CAD build for the part. Positions are in the model's coordinates, mm. Round coordinates to 2 decimals unless told otherwise and drop trailing zeros. Write each loop counter-clockwise with the first axis right and the second up, starting at its lowest first coordinate (ties: lowest second). Pieces come first, ordered by that corner, then holes. Notation, with made-up numbers: (41.5, 81) -> (67.5, 81) arc R14 cw to (67.5, 93) -> close; hole circle Ø8 at (-25, 60). An arc over 180 degrees is marked (long way). Put each result on its own line as item: value. Start each with the question number.
1. Flat gauge pins, fed straight in: P1, Ø8, axis at x = -3039.73, z = -145.15, coming from the +Y side; P2, Ø11.5, axis at x = -2919.73, z = -145.15, coming from the -Y side. Where does each tip first touch, or does it go through?
2. Drill centre lines: line 1 (X direction, y = 17.5, z = -35.5); line 2 (X direction, y = 20, z = -137); line 3 (Z direction, x = -3767.5, y = 2). Where is each one in solid material? Low to high. Write a range as from..to.
3. Saw through at A-A on z = -96. List the corners of the cut face in (x, y).
4. Saw through at B-B on x = -3637. List the corners of the cut face in (y, z).
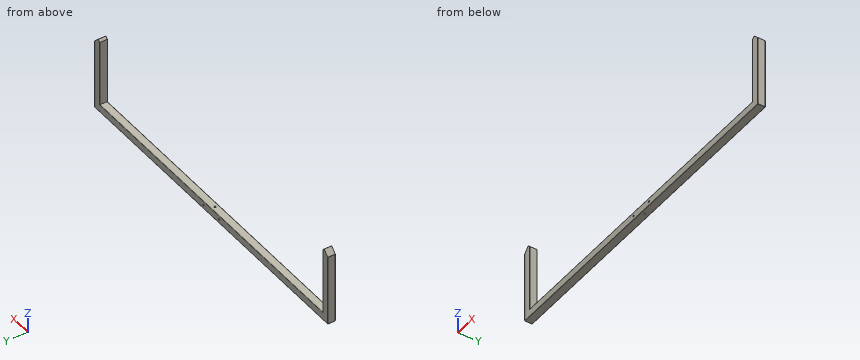
Autodesk Inventor part; units mm, degrees
ref_plane "YZ Plane" through (0, 0, 0) normal (1, 0, 0) x (0, 1, 0)
ref_plane "XZ Plane" through (0, 0, 0) normal (0, 1, 0) x (-1, 0, 0)
ref_plane "XY Plane" through (0, 0, 0) normal (0, 0, 1) x (1, 0, 0)
sketch "Sketch1" plane through (0, 0, 0) normal (0, 1, 0) x (-1, 0, 0)
  line L0 (3880.5632, 208.6837) -> (3853.3913, 235.9005)
  arc A0 (3880.5632, 208.6837) -> (3881.9735, 208.0967) centre (3881.9785, 210.0967) ccw
  line L1 (2078.8655, 206.2751) -> (2106.1695, 233.5659)
  arc A1 (2077.4795, 205.6899) -> (2078.8655, 206.2751) centre (2077.4516, 207.6897) ccw
  arc A2 (3883.0351, 262.7329) -> (3883.0378, 262.7357) centre (2978.5428, 1160.9837) ccw
  arc A3 (3881.9735, 261.6652) -> (3881.9774, 261.6692) centre (2978.5428, 1160.9837) ccw
  line L2 (2979.7274, -125.1538) -> (3881.9735, -125.1538)
  line L3 (3879.7274, -165.1538) -> (2079.7274, -165.1538)
  line L4 (2079.7274, -125.1538) -> (2979.7274, -125.1538)
  line L5 (3879.7274, -165.1538) -> (3881.9735, -165.1538)
  line L6 (2079.7274, -165.1538) -> (2077.4795, -165.1538)
  line L7 (2117.4795, -125.1538) -> (2077.4795, -125.1538)
  line L8 (2089.1735, -125.1538) -> (3870.2812, -125.1538)
  line L9 (2077.4795, 205.6899) -> (2077.4795, -165.1538)
  line L10 (2117.4795, 223.0557) -> (2117.4795, -125.1538)
  line L11 (3881.9735, 208.0967) -> (3881.9735, -165.1538)
  line L12 (3841.9735, 225.2347) -> (3841.9735, -125.1538)
  line L13 (3841.9735, -125.1538) -> (3881.9735, -125.1538)
  arc A4 (3841.9735, 225.2347) -> (3853.3913, 235.9005) centre (2978.5428, 1160.9837) ccw
  line L14 (2117.4795, 223.0557) -> (2106.1695, 233.5659)
  line L15 (3039.7274, -165.1538) -> (3039.7274, -145.1538)
  circle A5 centre (3039.7274, -145.1538) radius 5
  circle A6 centre (2919.7274, -145.1538) radius 5
  point P0 (0, 0)
  point P1 (2077.4509, 204.8613)
  point P2 (2106.1378, 233.5957)
  point P3 (2712.3694, -125.1538)
  dimension "d20" = 40
  dimension "d21" = 40
extrude "Extrusion1" add sketch "Sketch1" along normal blind 40 contours A0 L11 L2 L12 A4 L0 | L11 L5 L3 L6 L9 L7 L4 L2 | L4 L7 L9 A1 L1 L14 L10 | A5 | A6
fillet "Fillet1" radius 2 10 edges at (-3841.9735, 40, 50.0404) (-2979.7265, 40, -125.1538) (-3881.9735, 40, -145.1538) (-3881.9735, 40, 41.4714) (-2978.6034, 40, -165.1538) (-2077.4795, 40, 40.268) (-2077.4795, 40, -145.1538) (-2117.4795, 40, 48.9509) (-3841.9735, 0, 50.0404) (-2979.7265, 0, -125.1538)
fillet "Fillet2" radius 2 9 edges at (-2077.4795, 0, 40.268) (-2077.4795, 0, -145.1538) (-2978.6034, 0, -165.1538) (-2078.0653, 39.4142, -164.568) (-2077.4795, 19, -165.1538) (-3881.3877, 39.4142, -164.568) (-3881.9735, 19, -165.1538) (-3881.9735, 0, 41.4714) (-3881.9735, 0, -145.1538)
sketch "Sketch2" plane through (-2079.4795, 2, -165.1538) normal (0, 0, -1) x (-1, 0, 0)
  line L0 (0, 0) -> (0, 36)
  line L1 (0, 18) -> (1800.494, 18)
  line L2 (1800.494, 36) -> (1800.494, 0)
  circle A0 centre (900.247, 18) radius 5
  point P0 (-2079.4795, -2)
  dimension "d27" = 10
extrude "Extrusion2" cut sketch "Sketch2" against normal blind 50
extrude "Extrusion3" cut sketch "Sketch1" along normal blind 60 contours A5 | A6
properties part number "BASE_FUNDO_SUPORTE_LAMINA"
Return value:
1. P1: passes through
1. P2: stops at y = 0
2. line 1: x = -3881.97..-3841.97, -2117.48..-2077.48
2. line 2: x = -3881.97..-2984.73, -2974.73..-2077.48
2. line 3: z = -165.15..-125.15
3. outline: (-3881.97, 2) arc R2 ccw to (-3879.97, 0) -> (-3843.97, 0) arc R2 ccw to (-3841.97, 2) -> (-3841.97, 38) arc R2 ccw to (-3843.97, 40) -> (-3879.97, 40) arc R2 ccw to (-3881.97, 38) -> close; (-2117.48, 0) -> (-2079.48, 0) arc R2 ccw to (-2077.48, 2) -> (-2077.48, 38) arc R2 ccw to (-2079.48, 40) -> (-2115.48, 40) arc R2 ccw to (-2117.48, 38) -> close
4. outline: (0, -163.15) arc R2 ccw to (2, -165.15) -> (38, -165.15) arc R2 ccw to (40, -163.15) -> (40, -127.15) arc R2 ccw to (38, -125.15) -> (2, -125.15) arc R2 ccw to (0, -127.15) -> close
